Part print with two shaded views. Sizes in mm from the minimum x, y, z corner. A direction names the side the tool comes from. Coordinates: 2 decimals unless noted, no trailing zeros. Loops run counter-clockwise (first coordinate to the right, second up) from the corner with the lowest first, then second, coordinate; pieces in that order, holes last.
Item 1: Drill centre lines: line 1 along Y through (x, z) = (10.5, 2.5); line 2 along X through (y, z) = (5.75, 0.2); line 3 along Y through (x, z) = (17.5, 1.8). Where is each one in solid material? Low to high.
Item 2: Cut at B-B (z = 2). Count the separate pieces of the cut face and the enclosed holes in it, and give its area (3 significant figures).
Item 3: Cut at A-A (x = 11). List the corners of the cut face in (y, z).
Item 4: Cut at C-C (y = 4.5). List the corners of the cut face in (x, z), and give its area (3 significant figures).
Item 5: 3-axis set-ups, long thin cutter, end or side, ignore diameter. For the marked faces 1 and 2: which of +Z, -Z, +X, -X, +Y, -Y reach the whole face in a straight line?
Item 6: Cut at D-D (x = 16.25). List the corners of the cut face in (y, z), and give its area (3 significant figures).
Item 7: Flat gauge pins, fed straight in: pin 1 (1.5 mm diameter, centred on x = 2.5, z = 1.5, fed in from +Y); pin 2 (1 mm diameter, centred on y = 2.5, z = 1, fed in from +X). Where does each tip first touch, or does it go through?
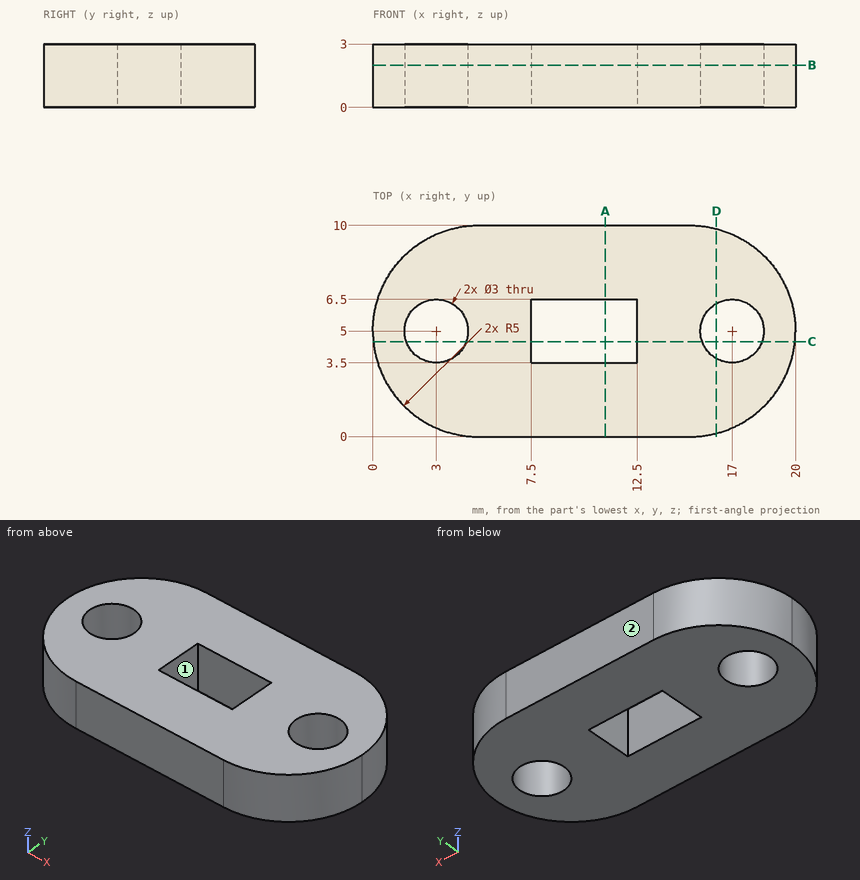
Filled sheet:
1. line 1: y = 0 to 3.5, 6.5 to 10
1. line 2: x = 0.06 to 1.7, 4.3 to 7.5, 12.5 to 15.7, 18.3 to 19.94
1. line 3: y = 0.67 to 3.59, 6.41 to 9.33
2. separate pieces: 1
2. enclosed holes: 3
2. area: 149 mm2
3. outline: (0, 0) - (3.5, 0) - (3.5, 3) - (0, 3) - close; (6.5, 0) - (10, 0) - (10, 3) - (6.5, 3) - close
4. outline: (0.03, 0) - (1.59, 0) - (1.59, 3) - (0.03, 3) - close; (4.41, 0) - (7.5, 0) - (7.5, 3) - (4.41, 3) - close; (12.5, 0) - (15.59, 0) - (15.59, 3) - (12.5, 3) - close; (18.41, 0) - (19.97, 0) - (19.97, 3) - (18.41, 3) - close
4. area: 27.9 mm2
5. face 1: +Z, -Z
5. face 2: +Z, -Z, +X, -X, +Y
6. outline: (0.16, 0) - (3.7, 0) - (3.7, 3) - (0.16, 3) - close; (6.3, 0) - (9.84, 0) - (9.84, 3) - (6.3, 3) - close
6. area: 21.3 mm2
7. pin 1: stops at y = 9.68
7. pin 2: stops at x = 19.58
